Check sheet for the modelled part. Datum: model origin and axes. Units: mm. Round coordinates to 2 decimals unless told otherwise and drop trailing zeros. Write each loop counter-clockwise with the first axis right and the second up, starting at its lowest first coordinate (ties: lowest second). Pieces come first, ordered by that corner, then holes. Notation, with made-up numbers: (47.5, 17) - (105.5, 17) arc R23 ccw to (105.5, 49) - close; hole circle Ø2 at (-26.75, -0.75). An arc over 180 degrees is marked (long way). Use one line per item in the form item = value. Start each with the question number.
1) Section check A-A (z = -286). Record the boundary of the cut face in (x, y), then the cut area to 3 significant figures.
2) Scan lines: probe 1 along Z at (x, y) = (558, -1.85); probe 2 along X at (y, z) = (-0.75, -379); probe 3 along X at (y, z) = (-2.3, 94.5). Record each from-to range of solid material in increasing order.
3) Gauge pin test, flat ends, axial feed: P1, Ø1.5, axis at y = -0.5, z = -342.5, coming from the -X side; P2, Ø2, axis at y = -2.5, z = -286.5, coming from the +X side. Record the tip position at first contact, or that the pin passes through.
4) Draft check along Z on faces 1 (the face through (584.063, -1.972, -358.071)), 2 (the face through (584, -4, -139)). Enter one of: +Z half, -Z half, draft (parallel to the pull), parting line (faces both ways), or undercut.
5) Section check B-B (x = 574.5). Count the separate pieces of the cut face and the enclosed holes in it, then the cut area to 3 significant figures.
from build123d import *

# Parameters (mm, degrees)
F0_R     = 15.6427266016
F0_R_2   = 12.0636627394
F1_DEPTH = 4


# Not quite as in the source:
# - a feature names something its author has since deleted; it is built from what else it names


with BuildPart() as f1:
    # F0 (on Front) → F1 (new body)
    with BuildSketch(Plane.XZ):
        with BuildLine():
            add(Edge.make_bspline(
                [(606.664408162, -6.3581708061), (610.2484126071, -61.6736918338), (611.0695149221, -116.339928141), (611.2557314215, -135.8581708061)],
                knots=[116.1389128405, 116.1389128405, 116.1389128405, 116.1389128405, 238.5747877883, 238.5747877883, 238.5747877883, 238.5747877883], degree=3))
            Line((606.664408162, -6.3581708061), (592.664408162, -6.3581708061))
            Line((592.664408162, -6.3581708061), (592.664408162, 1.1418291939))
            Line((592.664408162, 1.1418291939), (569.3247318268, 1.1418291939))
            Line((569.3247318268, 1.1418291939), (569.3247318268, -6.3581708061))
            Line((569.3247318268, -6.3581708061), (556.3105202547, -6.3581708061))
            add(Edge.make_bspline(
                [(556.3105202547, -6.3581708062), (556.3560675182, -46.8595634464), (556.3040983749, -91.0874507126), (556.321195241, -135.8581708062)],
                knots=[0.2731602209, 0.2731602209, 0.2731602209, 0.2731602209, 0.4883298337, 0.4883298337, 0.4883298337, 0.4883298337], degree=3))
            Line((556.321195241, -135.8581708061), (569.3247318268, -135.8581708061))
            Line((569.3247318268, -135.8581708061), (569.3247318268, -143.3581708061))
            Line((569.3247318268, -143.3581708061), (597.3095011307, -143.3581708061))
            Line((597.3095011307, -143.3581708061), (597.3095011307, -135.8581708061))
            Line((597.3095011307, -135.8581708061), (611.2557314215, -135.8581708061))
        make_face()
        with Locations((582.5758576393, -110.06578058)):
            Circle(F0_R, mode=Mode.SUBTRACT)
        with Locations((582.5758576393, -69.0548494458)):
            Circle(F0_R, mode=Mode.SUBTRACT)
        with Locations((582.5758576393, -30.3874015808)):
            Circle(F0_R, mode=Mode.SUBTRACT)
        with BuildLine():
            add(Edge.make_bspline(
                [(587.1910579171, 123.3613954191), (596.407592129, 101.4742246466), (602.1031854422, 55.9678384662), (605.6225226157, 8.6418291939)],
                knots=[0, 0, 0, 0, 105.0647905127, 105.0647905127, 105.0647905127, 105.0647905127], degree=3))
            Line((587.1910579171, 123.3613954191), (563.1910579171, 123.3613954191))
            Line((563.1910579171, 123.3613954191), (555.3247318268, 123.3613954191))
            add(Edge.make_bspline(
                [(555.3247318268, 123.3613954191), (555.9675431408, 93.7069693731), (556.2055580917, 53.8758795815), (556.2885566673, 8.6418291939)],
                knots=[0, 0, 0, 0, 0.2462769496, 0.2462769496, 0.2462769496, 0.2462769496], degree=3))
            Line((556.2885566673, 8.6418291939), (569.3247318268, 8.6418291939))
            Line((569.3247318268, 8.6418291939), (569.3247318268, 1.1418291939))
            Line((569.3247318268, 1.1418291939), (592.664408162, 1.1418291939))
            Line((592.664408162, 1.1418291939), (592.664408162, 8.6418291939))
            Line((592.664408162, 8.6418291939), (605.6225226157, 8.6418291939))
        make_face()
        with Locations((581.0006856918, 27.6772994548)):
            Circle(F0_R_2, mode=Mode.SUBTRACT)
        with Locations((575.1569867134, 95.7145318389)):
            Circle(F0_R_2, mode=Mode.SUBTRACT)
        with Locations((578.4962773323, 60.652397573)):
            Circle(F0_R_2, mode=Mode.SUBTRACT)
        with BuildLine():
            add(Edge.make_bspline(
                [(607.7513419726, -280.3581708061), (611.0463615473, -224.7368336409), (611.3157540895, -170.3281819541), (611.3171415076, -150.8581708061)],
                knots=[112.8825860344, 112.8825860344, 112.8825860344, 112.8825860344, 237.6045572103, 237.6045572103, 237.6045572103, 237.6045572103], degree=3))
            Line((611.3171415076, -150.8581708061), (611.3095011307, -150.8581708061))
            Line((611.3095011307, -150.8581708061), (597.3095011307, -150.8581708061))
            Line((597.3095011307, -150.8581708061), (597.3095011307, -143.3581708061))
            Line((597.3095011307, -143.3581708061), (569.3247318268, -143.3581708061))
            Line((569.3247318268, -143.3581708061), (569.3247318268, -150.8581708061))
            Line((569.3247318268, -150.8581708061), (556.3296648649, -150.8581708061))
            add(Edge.make_bspline(
                [(556.3296648649, -150.8581708062), (556.3627723501, -195.2400977423), (556.4619608218, -239.7521985209), (556.4380859402, -280.3581708061)],
                knots=[0.5123348883, 0.5123348883, 0.5123348883, 0.5123348883, 0.7252628697, 0.7252628697, 0.7252628697, 0.7252628697], degree=3))
            Line((556.4380859402, -280.3581708061), (569.3247318268, -280.3581708061))
            Line((569.3247318268, -280.3581708061), (569.3247318268, -287.8581708061))
            Line((569.3247318268, -287.8581708061), (569.3247318268, -295.3581708061))
            Line((569.3247318268, -295.3581708061), (556.4230475774, -295.3581708061))
            add(Edge.make_bspline(
                [(556.4230475774, -295.3581708061), (556.3560187283, -341.4793760002), (556.0897539461, -381.6099515969), (555.3247318268, -409.3581708061)],
                knots=[0.7518138312, 0.7518138312, 0.7518138312, 0.7518138312, 1, 1, 1, 1], degree=3))
            Line((555.3247318268, -409.3581708061), (556.8649172783, -409.3581708061))
            Line((556.8649172783, -409.3581708061), (589.3247318268, -409.3581708061))
            add(Edge.make_bspline(
                [(589.3247318268, -409.3581708061), (598.3171301483, -384.7473411865), (603.6401377777, -340.6568702112), (606.7877271908, -295.3581708061)],
                knots=[0, 0, 0, 0, 101.6745497642, 101.6745497642, 101.6745497642, 101.6745497642], degree=3))
            Line((606.7877271908, -295.3581708061), (605.6225226157, -295.3581708061))
            Line((605.6225226157, -295.3581708061), (593.664408162, -295.3581708061))
            Line((593.664408162, -295.3581708061), (593.664408162, -280.3581708061))
            Line((593.664408162, -280.3581708061), (606.664408162, -280.3581708061))
            Line((606.664408162, -280.3581708061), (607.7513419726, -280.3581708061))
        make_face()
        with Locations((575.1569867134, -382.4308734512)):
            Circle(F0_R_2, mode=Mode.SUBTRACT)
        with Locations((578.4962773323, -347.3687391853)):
            Circle(F0_R_2, mode=Mode.SUBTRACT)
        with Locations((581.0006856918, -314.3936410671)):
            Circle(F0_R_2, mode=Mode.SUBTRACT)
        with Locations((582.5758576393, -256.3289400315)):
            Circle(F0_R, mode=Mode.SUBTRACT)
        with Locations((582.5758576393, -217.6614921665)):
            Circle(F0_R, mode=Mode.SUBTRACT)
        with Locations((582.5758576393, -176.6505610322)):
            Circle(F0_R, mode=Mode.SUBTRACT)
    extrude(amount=F1_DEPTH)


solid = f1.part
Results are:
q1.outline = (569.32, -4) - (593.66, -4) - (593.66, 0) - (569.32, 0) - close
q1.area = 97.4 mm²
q2.probe_1 = -409.36 to -295.36, -280.36 to -150.86, -135.86 to -6.36, 8.64 to 123.36
q2.probe_2 = 555.92 to 563.59, 586.72 to 597.14
q2.probe_3 = 555.8 to 563.15, 587.16 to 595.27
q3.P1 = 556.25
q3.P2 = 593.66
q4.face_1 = undercut
q4.face_2 = draft
q5.separate_pieces = 13
q5.enclosed_holes = 0
q5.area = 950 mm²
